from build123d import *

# Parameters (mm, degrees)
SKETCH1_W           = 29
SKETCH1_H           = 14
SKETCH1_W_2         = 7
SKETCH1_H_2         = 8
SKETCH1_R           = 1.5
BOSS_EXTRUDE1_DEPTH = 2.5


with BuildPart() as part:
    # Sketch1 → Boss-Extrude1 (new body)
    with BuildSketch(Plane(origin=(0, 0, 0), x_dir=(1, 0, 0), z_dir=(0, 1, 0))):
        Rectangle(SKETCH1_W, SKETCH1_H)
        with Locations((-18, 0)):
            Rectangle(SKETCH1_W_2, SKETCH1_H_2)
        with Locations((-18, 0)):
            Circle(SKETCH1_R, mode=Mode.SUBTRACT)
        with Locations((18, 0)):
            Rectangle(SKETCH1_W_2, SKETCH1_H_2)
        with Locations((18, 0)):
            Circle(SKETCH1_R, mode=Mode.SUBTRACT)
    extrude(amount=BOSS_EXTRUDE1_DEPTH)


solid = part.part
Geometry: final body of the model. Coordinates: model frame, mm. A direction names the side the tool comes from. Coordinates: 2 decimals unless noted, no trailing zeros. Order: outer loops, then holes, each group sorted by start corner. A loop starts at its lowest first (then second) coordinate and runs counter-clockwise, first axis right, second up.
(1) Access query for faces 1 (the face through (21.5, 1, 0)), 2 (the face through (-18, 1, -4)), 3 (the face through (18, 1, -4)), 4 (the face through (18, 1, 4)), 5 (the face through (-14.5, 1, 6)). Directions: +Z, -Z, +X, -X, +Y, -Y. A direction counts if a zero-diameter tool reaches every point of the face in a straight line with its end or side. Return the directions, or none.
(2) Section query C-C (y = 1.05). Return the cut outline in (x, z), plus the area to 3 significant figures.
(3) Section query A-A (x = -18). Return the cut outline in (y, z), plus the area to 3 significant figures.
(4) Material intervals for probe 1 along X at (y, z) = (1.2, 0); probe 2 along Z at (x, y) = (18, 0.7); probe 3 along X at (y, z) = (2, -1), sorted ascending.
(5) Section query D-D (z = 6). Return the cut outline in (x, y), plus the area to 3 significant figures.
(6) First-contact query: pin 1 (1.2 mm diameter, centred on y = 1.5, z = 5.5, fed in from +X); pin 2 (1.2 mm diameter, centred on x = 18, y = 1.5, fed in from +Z); pin 3 (2.5 mm diameter, centred on x = 18, z = 0, fed in from +Y). Flat tips, straight axial feed; report the tip coordinate or a pass-through.
(7) Section query B-B (z = 0). Return the cut outline in (x, y).
(8) Draft query along X for faces 6 (the face through (-19.5, 1.23, -0.07)), 7 (the face through (14.5, 1, 6)), 8 (the face through (0, 0, 0)). Return one class per face: pulls with the +X half, pulls with the -X half, needs draft (parallel to the pull), parting line crosses it, or undercut.
Solution:
1. face 1: +Z, -Z, +X, +Y, -Y
1. face 2: -Z, -X, +Y, -Y
1. face 3: -Z, +X, +Y, -Y
1. face 4: +Z, +X, +Y, -Y
1. face 5: +Z, -X, +Y, -Y
2. outline: (-21.5, -4) - (-14.5, -4) - (-14.5, -7) - (14.5, -7) - (14.5, -4) - (21.5, -4) - (21.5, 4) - (14.5, 4) - (14.5, 7) - (-14.5, 7) - (-14.5, 4) - (-21.5, 4) - close; hole circle Ø3 at (-18, 0); hole circle Ø3 at (18, 0)
2. area: 504 mm2
3. outline: (0, -4) - (2.5, -4) - (2.5, -1.5) - (0, -1.5) - close; (0, 1.5) - (2.5, 1.5) - (2.5, 4) - (0, 4) - close
3. area: 12.5 mm2
4. probe 1: x = -21.5 to -19.5, -16.5 to 16.5, 19.5 to 21.5
4. probe 2: z = -4 to -1.5, 1.5 to 4
4. probe 3: x = -21.5 to -19.12, -16.88 to 16.88, 19.12 to 21.5
5. outline: (-14.5, 0) - (14.5, 0) - (14.5, 2.5) - (-14.5, 2.5) - close
5. area: 72.5 mm2
6. pin 1: stops at x = 14.5
6. pin 2: stops at z = 4
6. pin 3: passes through
7. outline: (-21.5, 0) - (-19.5, 0) - (-19.5, 2.5) - (-21.5, 2.5) - close; (-16.5, 0) - (16.5, 0) - (16.5, 2.5) - (-16.5, 2.5) - close; (19.5, 0) - (21.5, 0) - (21.5, 2.5) - (19.5, 2.5) - close
8. face 6: undercut
8. face 7: pulls with the +X half
8. face 8: needs draft
